from build123d import *

# Parameters (mm, degrees)
F1_DEPTH = 50.8
F2_R     = 9.525
F3_DEPTH = 6.35
F3_TAPER = 30


# Not quite as in the source:
# - a feature names something its author has since deleted; it is built from what else it names


with BuildPart() as f1:
    # F0 (on Right) → F1 (new body)
    with BuildSketch(Plane.YZ):
        Polygon((0, 304.8), (0, 0), (4.7625, 0), (4.7625, 301.6177992369), (72.4345492237, 329.6484798189), (70.3996203774, 333.9604775462), align=None)
    extrude(amount=F1_DEPTH)

    # F2 (on face) → F3 (join)
    with BuildSketch(Plane.XZ):
        with Locations((16.9333333333, 127)):
            Circle(F2_R)
        with Locations((33.8666666667, 50.8)):
            Circle(F2_R)
    extrude(amount=F3_DEPTH, taper=F3_TAPER)


solid = f1.part
For this review, take the finished solid that the model builds, in its own axes (mm). A direction names the side the tool comes from. Round coordinates to 2 decimals unless told otherwise and drop trailing zeros. Write each loop counter-clockwise with the first axis right and the second up, starting at its lowest first coordinate (ties: lowest second). Pieces come first, ordered by that corner, then holes. Notation, with made-up numbers: M 39.25,-17.5 L 84.25,-17.5 A33 cw 84.25,13.5 Z; hole C -11,70.25 d5. An arc over 180 degrees is marked long. Write item = value, one per line. Start each with the question number.
(1) We need section A-A (x = 47). Give the boundary of the cut face in (y, z), then the cut area to 3 significant figures.
(2) We need section B-B (z = 105). Give the boundary of the cut face in (x, y), then the cut area to 3 significant figures.
(3) For faces 1 (the face through (25, 4.762, 149)), 2 (the face through (50.8, 4, 192)), list the 3-axis set-ups (+Z, -Z, +X, -X, +Y, -Y) from which the entire face can be reached by the end or side of a thin tool; tool diameter is ignored.
(4) We need section C-C (y = 14). Give the boundary of the cut face in (x, z).
(5) Clearance check with flat-ended pins moving along their axes: pin 1 Ø4 at (x, y) = (22, 15.5) entering from -Z; pin 2 Ø1.5 at (x, z) = (11, 296.5) entering from -Y; pin 3 Ø5 at (x, z) = (18, 244) entering from +Y. State where each tip first meets the part, or that it passes through.
(6) For line 1 along Y through (x, z) = (10, 188.5); line 2 along Z through (x, y) = (21.5, 55.5); line 3 along Z through (x, y) = (15, 50), list the stretches that pass through material, from the lowest coordinate up.
Results found:
q1.outline = M 0,0 L 4.76,0 L 4.76,301.62 L 72.43,329.65 L 70.4,333.96 L 0,304.8 Z
q1.area = 1,800 mm²
q2.outline = M 0,0 L 50.8,0 L 50.8,4.76 L 0,4.76 Z
q2.area = 242 mm²
q3.face_1 = -Z, +X, -X, +Y
q3.face_2 = +Z, -Z, +X, +Y, -Y
q4.outline = M 0,305.44 L 50.8,305.44 L 50.8,310.6 L 0,310.6 Z
q5.pin_1 = 305.24
q5.pin_2 = 0
q5.pin_3 = 4.76
q6.line_1 = 0 to 4.76
q6.line_2 = 322.63 to 327.79
q6.line_3 = 320.36 to 325.51
